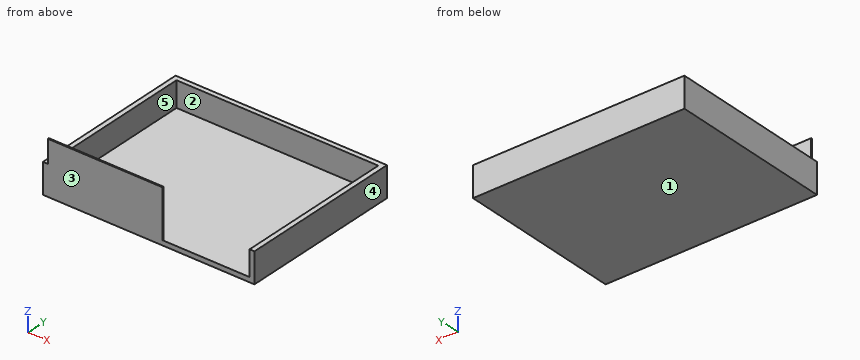
from build123d import *

# Parameters (mm, degrees)
F0_W     = 111.125
F0_H     = 86.36
F1_DEPTH = 15.875
F2_T     = -2.54
F3_W     = 60.325
F3_H     = 0.635
F4_DEPTH = 25.4


with BuildPart() as f1:
    # F0 (on Top) → F1 (new body)
    with BuildSketch(Plane.XY):
        Rectangle(F0_W, F0_H)
    extrude(amount=F1_DEPTH)

    # F2
    f2_openings = [f1.faces().sort_by_distance(p)[0] for p in [
        (0, 0, 15.875),
        (0, -43.18, 7.9375),
    ]]
    offset(amount=F2_T, openings=f2_openings)

    # F3 (on face) → F4 (join)
    with BuildSketch(Plane.XY.offset(2.54)):
        with Locations((-22.86, -42.8625)):
            Rectangle(F3_W, F3_H)
    extrude(amount=F4_DEPTH)


solid = f1.part
Geometry: final body of the model. Coordinates: model frame, mm. Face numbers are marked on the shaded views. A direction names the side the tool comes from. Give positions to 0.01 mm unless a question says otherwise; leave off trailing zeros. Write each loop counter-clockwise with the first axis right and the second up, starting at its lowest first coordinate (ties: lowest second). Pieces come first, ordered by that corner, then holes. Notation, with made-up numbers: (-3.5, 52.25) -> (19.5, 52.25) arc R21 cw to (19.5, 71.25) -> close; hole circle Ø5 at (87.25, 35.25). An arc over 180 degrees is marked (long way). Answer as a JSON object with one key per item and string values.
1. Mould query, pull axis Y, two halves, no side actions, for the marked faces 3, 4 and 5. Classes: pulls with the +Y half, pulls with the -Y half, needs draft (parallel to the pull), parting line crosses it, or undercut.
Ans:
{"face 3": "pulls with the -Y half", "face 4": "needs draft", "face 5": "undercut"}
2. Cut plane D-D on x = 16. Output: boundary loops of the cut face in (y, z) (3 decimals).
Ans:
{"outline": "(-43.18, 0) -> (43.18, 0) -> (43.18, 15.875) -> (40.64, 15.875) -> (40.64, 2.54) -> (-43.18, 2.54) -> close"}
3. Ray query, probe 1 along X at (y, z) = (24.5, 5.75); probe 2 along Y at (x, z) = (-43.5, 12.5) (3 decimals); probe 3 along Y at (x, z) = (-2.5, 21.5) (3 decimals). Return the intervals inside material, ascending. Write a range as from..to.
Ans:
{"probe 1": "x = -55.56..-53.02, 53.02..55.56", "probe 2": "y = -43.18..-42.545, 40.64..43.18", "probe 3": "y = -43.18..-42.545"}
4. Access query for the marked faces 1 and 2. Directions: +Z, -Z, +X, -X, +Y, -Y. A direction counts if a zero-diameter tool reaches every point of the face in a straight line with its end or side. Return the directions, or none.
Ans:
{"face 1": "-Z, +X, -X, +Y, -Y", "face 2": "+Z"}
5. Cut plane C-C on z = 12.5. Output: boundary loops of the cut face in (x, y) (1 decimal), and give its area (3 significant figures).
Ans:
{"outline": "(-55.6, -43.2) -> (7.3, -43.2) -> (7.3, -42.5) -> (-53, -42.5) -> (-53, 40.6) -> (53, 40.6) -> (53, -43.2) -> (55.6, -43.2) -> (55.6, 43.2) -> (-55.6, 43.2) -> close", "area": "746 mm^2"}
6. Cut plane B-B on y = 29. Output: boundary loops of the cut face in (x, z) (1 decimal), and give its area (3 significant figures).
Ans:
{"outline": "(-55.6, 0) -> (55.6, 0) -> (55.6, 15.9) -> (53, 15.9) -> (53, 2.5) -> (-53, 2.5) -> (-53, 15.9) -> (-55.6, 15.9) -> close", "area": "350 mm^2"}
7. Cut plane A-A on x = -25.5. Output: boundary loops of the cut face in (y, z) (3 decimals).
Ans:
{"outline": "(-43.18, 0) -> (43.18, 0) -> (43.18, 15.875) -> (40.64, 15.875) -> (40.64, 2.54) -> (-42.545, 2.54) -> (-42.545, 27.94) -> (-43.18, 27.94) -> close"}
8. Contact query for flat-ended pins moving along their axis: pin 1 (6 mm diameter, centred on x = -34.5, z = 19.5, fed in from +Y) (3 decimals); pin 2 (12 mm diameter, centred on x = -13.5, y = -6.5, fed in from +Z); pin 3 (0.7 mm diameter, centred on y = -43, z = 21.5, fed in from -X). Output: stop coordinate, or through.
Ans:
{"pin 1": "stops at y = -42.545", "pin 2": "stops at z = 2.54", "pin 3": "stops at x = -53.02"}
